from build123d import *

# Parameters (mm, degrees)
F1_DEPTH  = 25.4
F3_DEPTH  = 6.22
F7_DEPTH  = 25
F8_R      = 3.925
F9_DEPTH  = 15.3
F10_R     = 4
F11_DEPTH = 19.181
F12_R     = 4.75
F13_DEPTH = 25.401
F14_DEPTH = 25.401
F15_R     = 7.125
F16_DEPTH = 9.9
F17_DEPTH = 9.9


with BuildPart() as f1:
    # F0 (on Top) → F1 (new body)
    with BuildSketch(Plane.XY):
        with BuildLine():
            Line((0, -49.2), (0, 49.2))
            Line((0, 49.2), (-25.4, 49.2))
            Line((-25.4, 49.2), (-25.4, -13.5))
            ThreePointArc((-25.4, -13.5), (-26.571573, -16.328427), (-29.4, -17.5))
            Line((-29.4, -17.5), (-41.25, -17.5))
            Line((-41.25, -17.5), (-41.25, -49.2))
            Line((-41.25, -49.2), (0, -49.2))
        make_face()
    extrude(amount=F1_DEPTH)

    # F2 (on face) → F3 (cut)
    with BuildSketch(Plane.XY.offset(25.4)):
        with BuildLine():
            Line((0, 49.2), (-25.4, 49.2))
            Line((-25.4, 49.2), (-25.4, -4.7))
            Line((-25.4, -4.7), (-21.17, -4.7))
            ThreePointArc((-21.17, -4.7), (-19.755786, -4.114214), (-19.17, -2.7))
            Line((-19.17, -2.7), (-19.17, 20.5))
            ThreePointArc((-19.17, 20.5), (-18.584214, 21.914214), (-17.17, 22.5))
            Line((-17.17, 22.5), (0, 22.5))
            Line((0, 22.5), (0, 49.2))
        make_face()
    extrude(amount=-F3_DEPTH, mode=Mode.SUBTRACT)

    # F6 (on face) → F7 (cut)
    with BuildSketch(Plane(origin=(-16.581312, 1.684285, 0), x_dir=(0.101057, 0.994881, 0), z_dir=(0.994881, -0.101057, 0))):
        with BuildLine():
            Line((-19.283002, 9.4), (-19.283002, 30.4))
            Line((-19.283002, 30.4), (-56.146122, 30.4))
            Line((-56.146122, 30.4), (-56.146122, 6.4))
            Line((-56.146122, 6.4), (-22.283002, 6.4))
            ThreePointArc((-22.283002, 6.4), (-20.161682, 7.27868), (-19.283002, 9.4))
        make_face()
    extrude(amount=F7_DEPTH, mode=Mode.SUBTRACT)

    # F8 (on face) → F9 (cut)
    with BuildSketch(Plane(origin=(-16.581312, 1.684285, 0), x_dir=(0.101057, 0.994881, 0), z_dir=(0.994881, -0.101057, 0))):
        with Locations((-39.921122, 15.935)):
            Circle(F8_R)
    extrude(amount=-F9_DEPTH, mode=Mode.SUBTRACT)

    # F10 (on face) → F11 (cut, through all)
    with BuildSketch(Plane.XY.offset(19.18)):
        with Locations((-12.7, 36.45)):
            Circle(F10_R)
    extrude(amount=-F11_DEPTH, mode=Mode.SUBTRACT)

    # F12 (on face) → F13 (cut, through all)
    with BuildSketch(Plane.XY.offset(25.4)):
        with Locations((-9.52, 13.15)):
            Circle(F12_R)
    extrude(amount=-F13_DEPTH, mode=Mode.SUBTRACT)

    # F12 (on face) → F14 (cut, through all)
    with BuildSketch(Plane.XY.offset(25.4)):
        with Locations((-9.52, -9.65)):
            Circle(F12_R)
    extrude(amount=-F14_DEPTH, mode=Mode.SUBTRACT)

    # F15 (on face) → F16 (cut)
    with BuildSketch(Plane.XY.offset(25.4)):
        with Locations((-9.52, 13.15)):
            Circle(F15_R)
    extrude(amount=-F16_DEPTH, mode=Mode.SUBTRACT)

    # F15 (on face) → F17 (cut)
    with BuildSketch(Plane.XY.offset(25.4)):
        with Locations((-9.52, -9.65)):
            Circle(F15_R)
    extrude(amount=-F17_DEPTH, mode=Mode.SUBTRACT)


solid = f1.part
Can you work these out from the model? Positions are in its coordinate system, mm. A direction names the side the tool comes from. Round coordinates to 2 decimals unless told otherwise and drop trailing zeros. Write each loop counter-clockwise with the first axis right and the second up, starting at its lowest first coordinate (ties: lowest second). Pieces come first, ordered by that corner, then holes. Notation, with made-up numbers: M 5.25,89.25 L 34.25,89.25 A7 ccw 34.25,98.25 Z; hole C 55.25,82.5 d8. An arc over 180 degrees is marked long. Use a Markdown table: item, result.
Item 1: We'd pull the mould along Y, two halves only. Please class faces 1 (the face through (-5.69, -3.64, 20.52)), 2 (the face through (-19.77, -4.13, 22.33)), 3 (the face through (-41.25, -33, 13)): released by +Y, released by -Y, zero draft, split by the parting line, or undercut.
Found:
| item | result |
|---|---|
| face 1 | undercut |
| face 2 | released by +Y |
| face 3 | zero draft |
Item 2: I want a section at A-A (y = 36.45). List the corners of the cut face in (x, z) for me, and give its area (3 significant figures).
Found:
| item | result |
|---|---|
| outline | M -25.4,0 L -16.7,0 L -16.7,19.18 L -25.4,19.18 Z; M -8.7,0 L 0,0 L 0,19.18 L -8.7,19.18 Z |
| area | 334 mm2 |
Item 3: For pin 1 Ø8.5 at (x, y) = (-9.52, -9.65) entering from +Z; pin 2 Ø8 at (y, z) = (8, 15) entering from -X; pin 3 Ø12.5 at (x, y) = (-12, 34) entering from +Z; pin 4 Ø4 at (y, z) = (-24.5, 19.5) entering from +X, each with a flat end and sliding along its axis, tell me the tip position at first contact or that it passes through.
Found:
| item | result |
|---|---|
| pin 1 | passes through |
| pin 2 | stops at x = -25.4 |
| pin 3 | stops at z = 19.18 |
| pin 4 | stops at x = -19.04 |
Item 4: I want a section at B-B (y = 13.15). List the corners of the cut face in (x, z) for me (3 decimals), and give its area (3 significant figures).
Found:
| item | result |
|---|---|
| outline | M -25.4,0 L -14.27,0 L -14.27,15.5 L -16.645,15.5 L -16.645,25.4 L -19.17,25.4 L -19.17,19.18 L -25.4,19.18 Z; M -4.77,0 L 0,0 L 0,25.4 L -2.395,25.4 L -2.395,15.5 L -4.77,15.5 Z |
| area | 318 mm2 |
Item 5: I want a section at D-D (x = -12.7). State how many separate pieces and enclosed holes the cut face has, and give its area (3 significant figures).
Found:
| item | result |
|---|---|
| separate pieces | 4 |
| enclosed holes | 0 |
| area | 1,120 mm2 |
Item 6: I want a section at C-C (z = 13.5). List the corners of the cut face in (x, y) for me, and give its area (3 significant figures).
Found:
| item | result |
|---|---|
| outline | M -41.25,-49.2 L -21.75,-49.2 L -20.93,-41.1 L -36.15,-39.55 L -35.53,-33.42 L -20.3,-34.97 L -18.53,-17.5 L 0,-19.38 L 0,49.2 L -25.4,49.2 L -25.4,-13.5 A4 cw -29.4,-17.5 L -41.25,-17.5 Z; hole C -12.7,36.45 d8; hole C -9.52,-9.65 d9.5; hole C -9.52,13.15 d9.5 |
| area | 2,100 mm2 |
Item 7: If I drill on line 1 along Y through (x, z) = (-9.52, 22.75) (3 decimals); line 2 along Y through (x, z) = (-12.7, 13.5); line 3 along Y through (x, z) = (-9.52, 5.5), over which ranges is the centre line in solid material (lowest first)? Write a range as [from, to].
Found:
| item | result |
|---|---|
| line 1 | y = [-18.415, -16.775], [-2.525, 6.025], [20.275, 22.5] |
| line 2 | y = [-18.09, -13.18], [-6.12, 9.62], [16.68, 32.45], [40.45, 49.2] |
| line 3 | y = [-49.2, -14.4], [-4.9, 8.4], [17.9, 34.02], [38.88, 49.2] |
Item 8: Which directions (+Z, -Z, +X, -X, +Y, -Y) give clear straight access to the entire face, cutting with the end or side of a thin tool? Please do faces 4 (the face through (-10.448, 20.214, 20.519)), 5 (the face through (-23, -4.7, 22)), 6 (the face through (-35, -17.5, 13)).
Found:
| item | result |
|---|---|
| face 4 | +Z |
| face 5 | +Z, -X, +Y |
| face 6 | +Z, -Z, -X, +Y |
